Can you work these out from the model? Positions are in its coordinate system, mm. Face numbers are marked on the shaded views. A direction names the side the tool comes from. Give positions to 0.01 mm unless a question says otherwise; leave off trailing zeros. Write each loop counter-clockwise with the first axis right and the second up, starting at its lowest first coordinate (ties: lowest second). Pieces come first, ordered by that corner, then holes. Notation, with made-up numbers: (37, 24.5) -> (73, 24.5) arc R15 cw to (73, 29.5) -> close; hole circle Ø8 at (25.25, 18). An arc over 180 degrees is marked (long way). One line per item, written item: value.
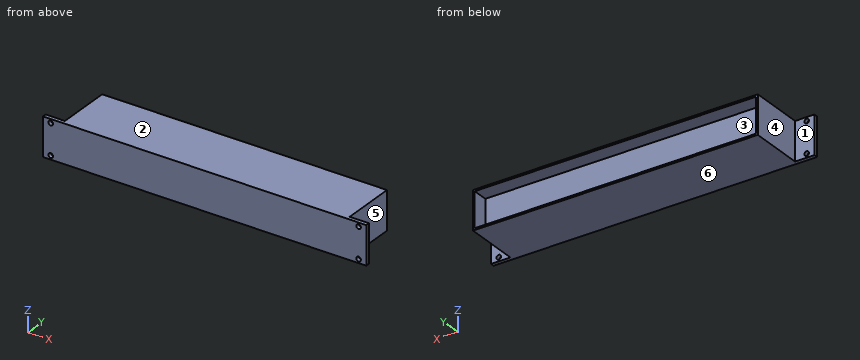
from build123d import *

# Parameters (mm, degrees)
SKETCH1_W           = 420
SKETCH1_H           = 50
SKETCH1_R           = 3
BOSS_EXTRUDE1_DEPTH = 75.75
SKETCH2_W           = 365.5
SKETCH2_H           = 45.5
CUT_EXTRUDE1_DEPTH  = 20
SKETCH3_W           = 25
SKETCH3_H           = 50
CUT_EXTRUDE2_DEPTH  = 70.75


with BuildPart() as part:
    # Sketch1 → Boss-Extrude1 (new body)
    with BuildSketch(Plane(origin=(0, 0, 0), x_dir=(1, 0, 0), z_dir=(0, 1, 0))):
        Rectangle(SKETCH1_W, SKETCH1_H)
        with Locations(Location((-200, -20, 0), (0, 0, 270))):
            Circle(SKETCH1_R, mode=Mode.SUBTRACT)
        with Locations(Location((200, -20, 0), (0, 0, 270))):
            Circle(SKETCH1_R, mode=Mode.SUBTRACT)
        with Locations(Location((-200, 20, 0), (0, 0, 270))):
            Circle(SKETCH1_R, mode=Mode.SUBTRACT)
        with Locations(Location((200, 20, 0), (0, 0, 90))):
            Circle(SKETCH1_R, mode=Mode.SUBTRACT)
    extrude(amount=BOSS_EXTRUDE1_DEPTH)

    # Sketch2 → Cut-Extrude1 (cut)
    with BuildSketch(Plane(origin=(0, 75.75, 0), x_dir=(1, 0, 0), z_dir=(0, 1, 0))):
        Rectangle(SKETCH2_W, SKETCH2_H)
    extrude(amount=-CUT_EXTRUDE1_DEPTH, mode=Mode.SUBTRACT)

    # Sketch3 → Cut-Extrude2 (cut)
    with BuildSketch(Plane(origin=(0, 75.75, 0), x_dir=(1, 0, 0), z_dir=(0, 1, 0))):
        with Locations((-197.5, 0)):
            Rectangle(SKETCH3_W, SKETCH3_H)
    cut_extrude2 = extrude(amount=-CUT_EXTRUDE2_DEPTH, mode=Mode.SUBTRACT)

    # Mirror1: Cut-Extrude2 across plane
    add(cut_extrude2.mirror(Plane(origin=(0, 0, 0), x_dir=(0, 0, 1), z_dir=(1, 0, 0))), mode=Mode.SUBTRACT)


solid = part.part
1) Will these pins go through, and if not, where does the flat tip stop? pin 1 (10 mm diameter, centred on y = 21, z = 14, fed in from -X); pin 2 (5.5 mm diameter, centred on x = -200, z = -20, fed in from -Y); pin 3 (7 mm diameter, centred on x = 200, z = -20, fed in from +Y); pin 4 (10 mm diameter, centred on y = 68, z = 10, fed in from +X).
Answer list:
pin 1: stops at x = -185
pin 2: passes through
pin 3: stops at y = 5
pin 4: stops at x = 185
2) For the marked faces 1 and 2, which set-ups out of +Z, -Z, +X, -X, +Y, -Y let a thin tool reach every point of the face, with its end or its side?
Answer list:
face 1: +Z, -Z, -X, +Y
face 2: +Z, +X, -X, +Y, -Y
3) I need wall thicknesses on L1, parallel to Z at x = 200, y = 3; L2, parallel to X at y = 2, z = 20; L3, parallel to Z at x = 115.5, y = 62.5. Which ranges of each line are inside material? Lowest first, please.
Answer list:
L1: z = -25 to -23, -17 to 17, 23 to 25
L2: x = -210 to -203, -197 to 197, 203 to 210
L3: z = -25 to -22.75, 22.75 to 25
4) If we section it at A-A (y = 62.5): Write out the boundary of the cut face in (x, z).
Answer list:
outline: (-185, -25) -> (185, -25) -> (185, 25) -> (-185, 25) -> close; hole (-182.75, -22.75) -> (182.75, -22.75) -> (182.75, 22.75) -> (-182.75, 22.75) -> close
5) We'd pull the mould along X, two halves only. Please class the marked faces 3, 4, 5 and 6: released by +X, released by -X, zero draft, split by the parting line, or undercut.
Answer list:
face 3: undercut
face 4: released by -X
face 5: released by +X
face 6: zero draft
6) If we section it at B-B (z = 1): Write out the boundary of the cut face in (x, y), and give its area (3 significant figures).
Answer list:
outline: (-210, 0) -> (210, 0) -> (210, 5) -> (185, 5) -> (185, 75.75) -> (182.75, 75.75) -> (182.75, 55.75) -> (-182.75, 55.75) -> (-182.75, 75.75) -> (-185, 75.75) -> (-185, 5) -> (-210, 5) -> close
area: 21,000 mm^2
7) If we section it at D-D (y = 30.5): Write out the boundary of the cut face in (x, z), and give its area (3 significant figures).
Answer list:
outline: (-185, -25) -> (185, -25) -> (185, 25) -> (-185, 25) -> close
area: 18,500 mm^2
8) If we section it at C-C (x = -56): Write out the boundary of the cut face in (y, z).
Answer list:
outline: (0, -25) -> (75.75, -25) -> (75.75, -22.75) -> (55.75, -22.75) -> (55.75, 22.75) -> (75.75, 22.75) -> (75.75, 25) -> (0, 25) -> close
